Check sheet for the modelled part. Datum: model origin and axes. Units: mm. Face numbers are marked on the shaded views. A direction names the side the tool comes from. Coordinates: 2 decimals unless noted, no trailing zeros. Write each loop counter-clockwise with the first axis right and the second up, starting at its lowest first coordinate (ties: lowest second). Pieces come first, ordered by that corner, then holes. Notation, with made-up numbers: (11.25, 71.25) -> (36.25, 71.25) arc R15 ccw to (36.25, 90.25) -> close; hole circle Ø11 at (-18, -31.75). An arc over 180 degrees is marked (long way). One line per item, written item: value. Start each with the question number.
1) Gauge pin test, flat ends, axial feed: P1, Ø2, axis at x = 1.5, z = 3, coming from the +Y side; P2, Ø5, axis at y = -8.5, z = -3.5, coming from the +X side; P3, Ø1, axis at y = -2, z = 2, coming from the +X side. Record the tip position at first contact, or that the pin passes through.
2) Sectioned sample at C-C on y = 0. Enter the section's corners in (x, z), plus the area to 3 significant figures.
3) Sectioned sample at D-D on x = 4.5. Enter the section's corners in (y, z).
4) Draft check along X on the marked faces 3, 4 and 5. Enter one of: +X half, -X half, draft (parallel to the pull), parting line (faces both ways), or undercut.
5) Set-up check for the marked faces 1 and 2: record each of +Z, -Z, +X, -X, +Y, -Y from which the full face is reachable in a straight line by a thin tool's end or side.
6) Sectioned sample at B-B on z = -0.5. Enter the section's corners in (x, y).
7) Scan lines: line 1 along Y through (x, z) = (-4.5, -1.2); line 2 along Z through (x, y) = (2.5, 7.25); line 3 along Z through (x, y) = (0, -5.5). Record each from-to range of solid material in increasing order. Write a range as [from, to].
8) Sectioned sample at A-A on x = 0. Enter the section's corners in (y, z), plus the area to 3 significant figures.
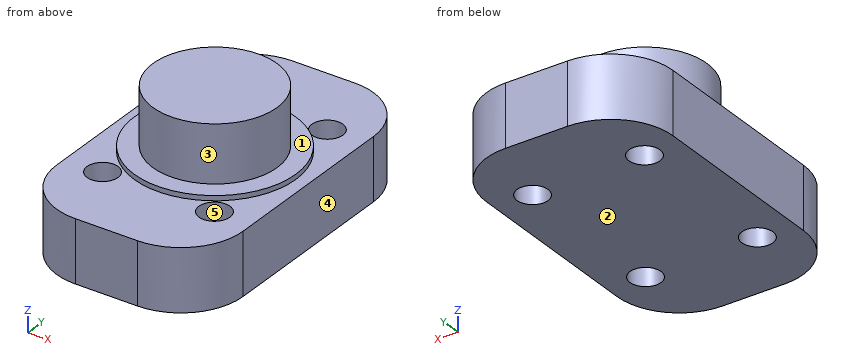
```python
from build123d import *

# Parameters (mm, degrees)
SKETCH_1_W      = 15
SKETCH_1_H      = 25
EXTRUDE_1_DEPTH = 5
SKETCH_1_3_R    = 6.5
EXTRUDE_2_DEPTH = 0.4
SKETCH_1_4_R    = 5
EXTRUDE_3_DEPTH = 5
M3X0_5_1_D      = 2.5
FILLET_1_R      = 5


with BuildPart() as part:
    # ｽｹｯﾁ1 → ﾎﾞｽ - 押し出し1 (new body)
    with BuildSketch(Plane.XY):
        Rectangle(SKETCH_1_W, SKETCH_1_H)
    extrude(amount=-EXTRUDE_1_DEPTH)

    # ｽｹｯﾁ1<3> → ﾎﾞｽ - 押し出し2 (add)
    with BuildSketch(Plane.XY):
        Circle(SKETCH_1_3_R)
    extrude(amount=EXTRUDE_2_DEPTH)

    # ｽｹｯﾁ1<4> → ﾎﾞｽ - 押し出し3 (add)
    with BuildSketch(Plane.XY):
        Circle(SKETCH_1_4_R)
    extrude(amount=EXTRUDE_3_DEPTH)

    # M3x0.5 ねじ穴用ねじ下穴ﾄﾞﾘﾙ1 (through all)
    with Locations(Plane(origin=(-4.5, 6.5, 0), x_dir=(1, 0, 0), z_dir=(0, 0, 1))):
        with Locations((0, 0), (9, 0), (9, -13), (0, -13)):
            Hole(M3X0_5_1_D / 2)

    # ﾌｨﾚｯﾄ1
    fillet_1_edges = [part.edges().sort_by_distance(p)[0] for p in [
        (-7.5, 12.5, -2.5),
        (7.5, 12.5, -2.5),
        (7.5, -12.5, -2.5),
        (-7.5, -12.5, -2.5),
    ]]
    fillet(fillet_1_edges, radius=FILLET_1_R)


solid = part.part
```
Answers:
1. P1: stops at y = 4.97
1. P2: stops at x = 7.5
1. P3: stops at x = 4.77
2. outline: (-7.5, -5) -> (7.5, -5) -> (7.5, 0) -> (6.5, 0) -> (6.5, 0.4) -> (5, 0.4) -> (5, 5) -> (-5, 5) -> (-5, 0.4) -> (-6.5, 0.4) -> (-6.5, 0) -> (-7.5, 0) -> close
2. area: 126 mm2
3. outline: (-12.08, -5) -> (-7.75, -5) -> (-7.75, 0) -> (-12.08, 0) -> close; (-5.25, -5) -> (5.25, -5) -> (5.25, 0) -> (4.69, 0) -> (4.69, 0.4) -> (2.18, 0.4) -> (2.18, 5) -> (-2.18, 5) -> (-2.18, 0.4) -> (-4.69, 0.4) -> (-4.69, 0) -> (-5.25, 0) -> close; (7.75, -5) -> (12.08, -5) -> (12.08, 0) -> (7.75, 0) -> close
4. face 3: parting line
4. face 4: +X half
4. face 5: undercut
5. face 1: +Z
5. face 2: -Z, +X, -X, +Y, -Y
6. outline: (-7.5, -7.5) arc R5 ccw to (-2.5, -12.5) -> (2.5, -12.5) arc R5 ccw to (7.5, -7.5) -> (7.5, 7.5) arc R5 ccw to (2.5, 12.5) -> (-2.5, 12.5) arc R5 ccw to (-7.5, 7.5) -> close; hole circle Ø2.5 at (-4.5, -6.5); hole circle Ø2.5 at (-4.5, 6.5); hole circle Ø2.5 at (4.5, -6.5); hole circle Ø2.5 at (4.5, 6.5)
7. line 1: y = [-12.08, -7.75], [-5.25, 5.25], [7.75, 12.08]
7. line 2: z = [-5, 0]
7. line 3: z = [-5, 0.4]
8. outline: (-12.5, -5) -> (12.5, -5) -> (12.5, 0) -> (6.5, 0) -> (6.5, 0.4) -> (5, 0.4) -> (5, 5) -> (-5, 5) -> (-5, 0.4) -> (-6.5, 0.4) -> (-6.5, 0) -> (-12.5, 0) -> close
8. area: 176 mm2
